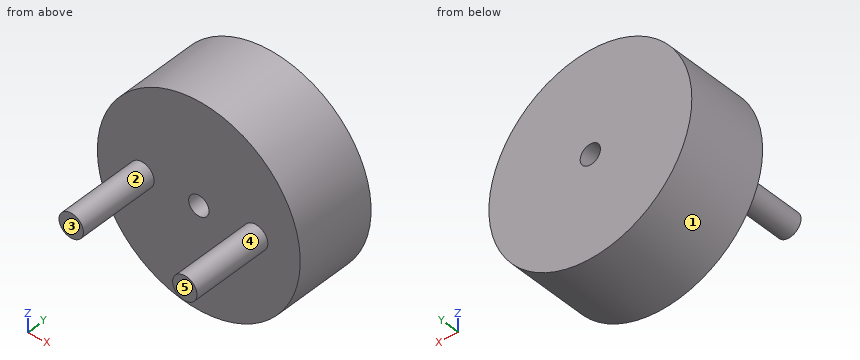
Autodesk Inventor part; units mm, degrees
ref_plane "YZ Plane" through (0, 0, 0) normal (1, 0, 0) x (0, 1, 0)
ref_plane "XZ Plane" through (0, 0, 0) normal (0, 1, 0) x (-1, 0, 0)
ref_plane "XY Plane" through (0, 0, 0) normal (0, 0, 1) x (1, 0, 0)
sketch "Sketch1" plane through (0, 0, 0) normal (0, 1, 0) x (-1, 0, 0)
  circle A0 centre (0, 0) radius 12.5
  circle A1 centre (0, 0) radius 1.25
  dimension "d0" = 25
  dimension "d1" = 2.5
extrude "Extrusion1" add sketch "Sketch1" along normal blind 10
sketch "Sketch2" plane through (0, 0, 0) normal (0, -1, 0) x (1, 0, 0)
  circle A0 centre (-7, 0) radius 1.5
  circle A1 centre (7, 0) radius 1.5
  point P0 (0, 0)
  dimension "d4" = 3
  dimension "d5" = 3
  dimension "d6" = 7
  dimension "d7" = 7
extrude "Extrusion2" add sketch "Sketch2" along normal blind 10
properties part number "buzz"
The listing builds one solid part. Answer for the finished solid, in the listing's coordinates (mm). Face numbers are marked on the shaded views. A direction names the side the tool comes from. Coordinates: 2 decimals unless noted, no trailing zeros. Write each loop counter-clockwise with the first axis right and the second up, starting at its lowest first coordinate (ties: lowest second). Pieces come first, ordered by that corner, then holes. Notation, with made-up numbers: M -15.5,28.25 L 38.5,28.25 A24 cw 38.5,64.25 Z; hole C 12,25.25 d7. An arc over 180 degrees is marked long. Use a Markdown table: item, result. Add a question column.
1. Straight lines are drawn through the part: line 1 along Z through (x, y) = (0, 4.25); line 2 along Y through (x, z) = (5.5, 2.5); line 3 along Z through (x, y) = (-7, -2.75). For each, find the intervals that lie inside material, in ascending order. Write a range as [from, to].
2. For a pull along X with two mould halves and no side action, classify the marked faces 1, 2 and 3 as +X half, -X half, draft (parallel to the pull), parting line (faces both ways), or undercut.
3. Section D-D (y = 1.5) is taken. Give the vertices of the cut face in (x, z), plus the area to 3 significant figures.
4. Which of the six approach directions +Z, -Z, +X, -X, +Y, -Y give full straight-line access (tool end or side, diameter ignored) to the marked faces 4 and 5?
5. Section C-C (y = -6.25) is taken. Give the vertices of the cut face in (x, z), plus the area to 3 significant figures.
6. Section B-B (z = -0.75) is taken. Give the vertices of the cut face in (x, y), plus the area to 3 significant figures.
7. Section A-A (x = 0) is taken. Give the vertices of the cut face in (y, z).
8. Given P1, Ø4, axis at x = -4, y = 2.5, coming from the -Z side; P2, Ø1, axis at x = 3, z = -2, coming from the -Y side; P3, Ø10, axis at x = 5.5, y = -3, coming from the +Z side, each flat-ended and moving along its own axis, determine where each tip first touches the part or whether it passes through.
Data:
| question | item | result |
|---|---|---|
| 1 | line 1 | z = [-12.5, -1.25], [1.25, 12.5] |
| 1 | line 2 | y = [0, 10] |
| 1 | line 3 | z = [-1.5, 1.5] |
| 2 | face 1 | parting line |
| 2 | face 2 | undercut |
| 2 | face 3 | draft |
| 3 | outline | C 0,0 d25; hole C 0,0 d2.5 |
| 3 | area | 486 mm2 |
| 4 | face 4 | -Y |
| 4 | face 5 | +Z, -Z, +X, -X, -Y |
| 5 | outline | C -7,0 d3; C 7,0 d3 |
| 5 | area | 14.1 mm2 |
| 6 | outline | M -12.48,0 L -8.3,0 L -8.3,-10 L -5.7,-10 L -5.7,0 L -1,0 L -1,10 L -12.48,10 Z; M 1,0 L 5.7,0 L 5.7,-10 L 8.3,-10 L 8.3,0 L 12.48,0 L 12.48,10 L 1,10 Z |
| 6 | area | 282 mm2 |
| 7 | outline | M 0,-12.5 L 10,-12.5 L 10,-1.25 L 0,-1.25 Z; M 0,1.25 L 10,1.25 L 10,12.5 L 0,12.5 Z |
| 8 | P1 | stops at z = -12.34 |
| 8 | P2 | stops at y = 0 |
| 8 | P3 | stops at z = 12.41 |
